Source: CAD feature listing. Evaluate the final solid. Frame: model axes, mm. Face numbers are marked on the shaded views. A direction names the side the tool comes from. Coordinates: 2 decimals unless noted, no trailing zeros. Order: outer loops, then holes, each group sorted by start corner. A loop starts at its lowest first (then second) coordinate and runs counter-clockwise, first axis right, second up. Notation, with made-up numbers: (60.5, 41) - (111.5, 41) arc R16 ccw to (111.5, 62) - close; hole circle Ø11 at (-4, -9.75). An arc over 180 degrees is marked (long way). One line per question, with ' | ' between items.
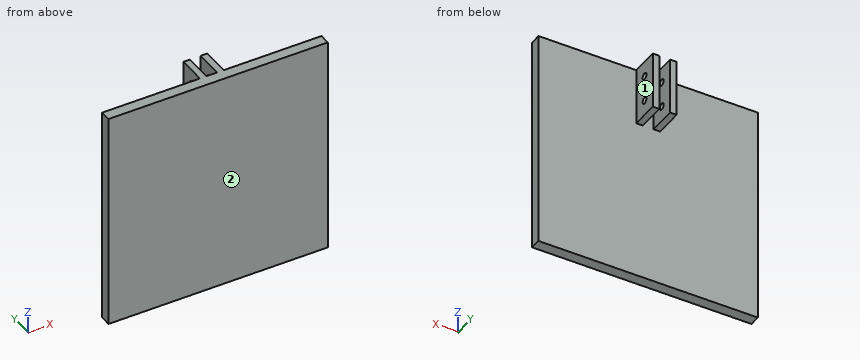
from build123d import *

# Parameters (mm, degrees)
SKETCH1_W           = 101.6
SKETCH1_H           = 101.6
BOSS_EXTRUDE1_DEPTH = 5
SKETCH2_W           = 3
SKETCH2_H           = 26.31
BOSS_EXTRUDE2_DEPTH = 13
SKETCH3_R           = 1.5
CUT_EXTRUDE1_DEPTH  = 13


with BuildPart() as part:
    # Sketch1 → Boss-Extrude1 (new body)
    with BuildSketch(Plane(origin=(0, 0, 0), x_dir=(1, 0, 0), z_dir=(0, 1, 0))):
        Rectangle(SKETCH1_W, SKETCH1_H)
    extrude(amount=BOSS_EXTRUDE1_DEPTH)

    # Sketch2 → Boss-Extrude2 (add)
    with BuildSketch(Plane(origin=(0, 5, 0), x_dir=(1, 0, 0), z_dir=(0, 1, 0))):
        with Locations((-4, -37.645)):
            Rectangle(SKETCH2_W, SKETCH2_H)
        with Locations((4, -37.645)):
            Rectangle(SKETCH2_W, SKETCH2_H)
    extrude(amount=BOSS_EXTRUDE2_DEPTH)

    # Sketch3 → Cut-Extrude1 (cut)
    with BuildSketch(Plane(origin=(5.5, 0, 0), x_dir=(0, 0, -1), z_dir=(1, 0, 0))):
        with Locations((-43.63, 11.5)):
            Circle(SKETCH3_R)
        with Locations((-31.66, 11.5)):
            Circle(SKETCH3_R)
    extrude(amount=-CUT_EXTRUDE1_DEPTH, mode=Mode.SUBTRACT)


solid = part.part
(1) Cut plane D-D (x = 13). Return the cut outline in (y, z), and give its area (3 significant figures).
Taken from the geometry:
outline: (0, -50.8) - (5, -50.8) - (5, 50.8) - (0, 50.8) - close | area: 508 mm²
(2) Cut plane B-B (y = 11.5). Return the cut outline in (x, z), and give its area (3 significant figures).
Taken from the geometry:
outline: (-5.5, 24.49) - (-2.5, 24.49) - (-2.5, 30.16) - (-5.5, 30.16) - close; (-5.5, 33.16) - (-2.5, 33.16) - (-2.5, 42.13) - (-5.5, 42.13) - close; (-5.5, 45.13) - (-2.5, 45.13) - (-2.5, 50.8) - (-5.5, 50.8) - close; (2.5, 24.49) - (5.5, 24.49) - (5.5, 30.16) - (2.5, 30.16) - close; (2.5, 33.16) - (5.5, 33.16) - (5.5, 42.13) - (2.5, 42.13) - close; (2.5, 45.13) - (5.5, 45.13) - (5.5, 50.8) - (2.5, 50.8) - close | area: 122 mm²
(3) Cut plane A-A (z = 43.63). Return the cut outline in (x, y).
Taken from the geometry:
outline: (-50.8, 0) - (50.8, 0) - (50.8, 5) - (5.5, 5) - (5.5, 10) - (2.5, 10) - (2.5, 5) - (-2.5, 5) - (-2.5, 10) - (-5.5, 10) - (-5.5, 5) - (-50.8, 5) - close; (-5.5, 13) - (-2.5, 13) - (-2.5, 18) - (-5.5, 18) - close; (2.5, 13) - (5.5, 13) - (5.5, 18) - (2.5, 18) - close
(4) Pin query (flat end, axial travel): P1, Ø4, axis at y = 11.5, z = 31.66, coming from the -X side; P2, Ø5, axis at x = 6, z = -18.5, coming from the +Y side; P3, Ø4, axis at y = 11.5, z = 43.63, coming from the +X side; P4, Ø1.8, axis at y = 11.5, z = 43.63, coming from the +X side. Return the tip coordinate at first contact, or that it passes through.
Taken from the geometry:
P1: stops at x = -5.5 | P2: stops at y = 5 | P3: stops at x = 5.5 | P4: passes through
(5) Material intervals for L1, parallel to Y at x = -3.2, z = 31.66; L2, parallel to Y at x = 6.5, z = -28.5, sorted ascending. Write a range as from..to.
Taken from the geometry:
L1: y = 0..10, 13..18 | L2: y = 0..5
(6) Set-up query: the marked faces 1 and 2. Return all of +Z, -Z, +X, -X, +Y, -Y with unobstructed straight access to the full face (end or side cutting, diameter ignored); none if empty.
Taken from the geometry:
face 1: +Z, -Z, +X, +Y | face 2: +Z, -Z, +X, -X, -Y
(7) Cut plane C-C (z = -31). Return the cut outline in (x, y), and give its area (3 significant figures).
Taken from the geometry:
outline: (-50.8, 0) - (50.8, 0) - (50.8, 5) - (-50.8, 5) - close | area: 508 mm²
